```python
from build123d import *

# Parameters (mm, degrees)
SKETCH1_W            = 32
SKETCH1_H            = 110
BOSS_EXTRUDE1_DEPTH  = 3
SKETCH2_W            = 6
SKETCH2_H            = 69
BOSS_EXTRUDE2_DEPTH  = 30
CUT_EXTRUDE1_DEPTH   = 69
FILLET1_R            = 10
FILLET1_OF_MIRROR1_R = 10
SKETCH4_W            = 15
SKETCH4_H            = 15
SKETCH4_W_2          = 8
SKETCH4_H_2          = 8
CUT_EXTRUDE2_DEPTH   = 117.456000275


with BuildPart() as part:
    # Sketch1 → Boss-Extrude1 (new body)
    with BuildSketch(Plane(origin=(0, 0, 0), x_dir=(1, 0, 0), z_dir=(0, 1, 0))):
        with Locations((16, 55)):
            Rectangle(SKETCH1_W, SKETCH1_H)
    boss_extrude1 = extrude(amount=BOSS_EXTRUDE1_DEPTH)

    # Sketch2 → Boss-Extrude2 (add)
    with BuildSketch(Plane(origin=(0, 3, 0), x_dir=(1, 0, 0), z_dir=(0, 1, 0))):
        Polygon((0, 3), (0, 0), (32, 0), (32, 3), (26, 3), align=None)
        with Locations((29, 37.5)):
            Rectangle(SKETCH2_W, SKETCH2_H)
    boss_extrude2 = extrude(amount=BOSS_EXTRUDE2_DEPTH)

    # Sketch3 → Cut-Extrude1 (cut)
    with BuildSketch(Plane(origin=(0, 0, -72), x_dir=(-1, 0, 0), z_dir=(0, 0, -1))):
        Polygon((-26, 32), (-28, 30), (-28, 29), (-26, 29), align=None)
    cut_extrude1 = extrude(amount=-CUT_EXTRUDE1_DEPTH, mode=Mode.SUBTRACT)

    # Fillet1
    fillet1_edges = [part.edges().sort_by_distance(p)[0] for p in [
        (32, 1.5, -110),
    ]]
    fillet(fillet1_edges, radius=FILLET1_R)

    # Mirror1: Boss-Extrude1, Boss-Extrude2, Cut-Extrude1 across plane
    add(boss_extrude1.mirror(Plane(origin=(0, 3, 0), x_dir=(0, 0, 1), z_dir=(1, 0, 0))))
    add(boss_extrude2.mirror(Plane(origin=(0, 3, 0), x_dir=(0, 0, 1), z_dir=(1, 0, 0))))
    add(cut_extrude1.mirror(Plane(origin=(0, 3, 0), x_dir=(0, 0, 1), z_dir=(1, 0, 0))), mode=Mode.SUBTRACT)

    # Fillet1 of Mirror1
    fillet1_of_mirror1_edges = [part.edges().sort_by_distance(p)[0] for p in [
        (-32, 1.5, -110),
    ]]
    fillet(fillet1_of_mirror1_edges, radius=FILLET1_OF_MIRROR1_R)

    # Sketch4 → Cut-Extrude2 (cut, through all)
    with BuildSketch(Plane(origin=(0, 0, -3), x_dir=(-1, 0, 0), z_dir=(0, 0, -1))):
        with Locations((8.5, 20.5)):
            Rectangle(SKETCH4_W, SKETCH4_H)
        with Locations((-8, 7)):
            Rectangle(SKETCH4_W_2, SKETCH4_H_2)
    extrude(amount=-CUT_EXTRUDE2_DEPTH, mode=Mode.SUBTRACT)


solid = part.part
```
Here's how the part is built. I have some questions about the finished solid (model axes, mm). A direction names the side the tool comes from. Give positions to 0.01 mm unless a question says otherwise; leave off trailing zeros. Loops run counter-clockwise (first coordinate to the right, second up) from the corner with the lowest first, then second, coordinate; pieces in that order, holes last. Notation, with made-up numbers: M 10,36.25 L 63,36.25 A25 ccw 63,56.25 Z; hole C -17.75,76 d6. An arc over 180 degrees is marked long. Use one line per item in the form item = value. Start each with the question number.
Q1. If we section it at A-A (y = 9.5): Write out the boundary of the cut face in (x, z), then the cut area to 3 significant figures.
Q2. If we section it at D-D (x = -18): Write out the boundary of the cut face in (y, z).
Q3. Thinking about a two-plate mould opening in X: for faces 1 (the flat face through (4, 7, -2)), 2 (the flat face through (0, 0, -56)), 3 (the flat face through (-32, 16, -38)), which applies, +X half, -X half, draft (parallel to the pull), parting line (faces both ways), or undercut?
Q4. Which directions (+Z, -Z, +X, -X, +Y, -Y) give clear straight access to the entire face, cutting with the end or side of a thin tool? Please do faces 4 (the flat face through (32, 16, -38)), 5 (the flat face through (27, 31, -38)), 6 (the flat face through (29, 18, -72)), 7 (the flat face through (8, 11, -2)).
Q5. Will these pins go through, and if not, where does the flat tip stop? pin 1 Ø10 at (x, z) = (-17, -64.5) entering from +Y; pin 2 Ø8 at (x, y) = (9, 12) entering from -Z.
Q6. If we section it at C-C (z = -54): Write out the boundary of the cut face in (x, y).
Q7. I need wall thicknesses on line 1 along X through (y, z) = (7, -11); line 2 along Y through (x, z) = (3.5, -27); line 3 along Z through (x, y) = (21.5, 11). Which ranges of each line are inside material? Lowest first, please.
Q8. If we section it at B-B (x = -5): Write out the boundary of the cut face in (y, z), then the cut area to 3 significant figures.
Taken from the geometry:
q1.outline = M -32,-72 L -26,-72 L -26,-3 L 4,-3 L 4,0 L -32,0 Z; M 12,-3 L 26,-3 L 26,-72 L 32,-72 L 32,0 L 12,0 Z
q1.area = 996 mm^2
q2.outline = M 0,-110 L 3,-110 L 3,-3 L 33,-3 L 33,0 L 0,0 Z
q3.face_1 = undercut
q3.face_2 = draft
q3.face_3 = -X half
q4.face_4 = +Z, -Z, +X, +Y, -Y
q4.face_5 = -Z
q4.face_6 = -Z, +X, -X, +Y
q4.face_7 = +Z, -Z
q5.pin_1 = 3
q5.pin_2 = -3
q6.outline = M -32,0 L 32,0 L 32,33 L 26,33 L 26,32 L 28,30 L 28,29 L 26,29 L 26,3 L -26,3 L -26,29 L -28,29 L -28,30 L -26,32 L -26,33 L -32,33 Z
q7.line_1 = -32 to -26, 26 to 32
q7.line_2 = 0 to 3
q7.line_3 = -3 to 0
q8.outline = M 0,-110 L 3,-110 L 3,-3 L 13,-3 L 13,0 L 0,0 Z; M 28,-3 L 33,-3 L 33,0 L 28,0 Z
q8.area = 375 mm^2
